Source: CAD feature listing. Evaluate the final solid. Frame: model axes, mm. A direction names the side the tool comes from. Give positions to 0.01 mm unless a question says otherwise; leave off trailing zeros. Order: outer loops, then holes, each group sorted by start corner. A loop starts at its lowest first (then second) coordinate and runs counter-clockwise, first axis right, second up. Notation, with made-up numbers: M 57,42.5 L 93,42.5 A30 ccw 93,70.5 Z; hole C -0.75,31.5 d9. An arc over 180 degrees is marked long. Use CSV: the item, a comma, the result in double quotes. Start each with the question number.
1. Reachability of faces 4 (the cylindrical face through (56.99, 1.52, -29.15)), 5 (the flat face through (-10, 1, -25)) from +Z, -Z, +X, -X, +Y, -Y: full face, straight path, thin tool, end or side. Return the list, or none.
2. Section query A-A, the plane y = 2.15. Return the cut outline in (x, z).
3. Line query: line 1 along X through (y, z) = (2.4, -17.5); line 2 along X through (y, z) = (2.35, -22); line 3 along Z through (x, y) = (-0.5, 1.25). Output: solid intervals per line, ascending. Write a range as [from, to].
4. Section query B-B, the plane x = -41. Return the cut outline in (y, z).
5. Mould query, pull axis X, two halves, no side actions, for faces 1 (the flat face through (0, 1, 32)), 2 (the flat face through (0, 1, -12)), 3 (the cylindrical face through (31.35, 1.48, 30.05)). Classes: released by +X, released by -X, zero draft, split by the parting line, or undercut.
6. Pin query (flat end, axial travel): P1, Ø1.5, axis at x = 29.5, z = 16, coming from the -Y side; P2, Ø0.9, axis at y = 1, z = -25, coming from the +X side; P3, Ø2.5, axis at x = 50, z = -22, coming from the +Y side. Return the tip coordinate at first contact, or that it passes through.
from build123d import *

# Parameters (mm, degrees)
SKETCH_1_W          = 120
SKETCH_1_H          = 64
EXTRUDE_1_DEPTH     = 3
SKETCH_2_R          = 1.5
CUT_EXTRUDE_1_DEPTH = 3
FILLET_1_R          = 10
SKETCH_3_W          = 20
SKETCH_3_H          = 20
CUT_EXTRUDE_2_DEPTH = 3
SKETCH_4_R          = 26
CUT_EXTRUDE_3_DEPTH = 3
FILLET_2_R          = 5
FILLET_3_R          = 10
FILLET_4_R          = 10
SKETCH_6_R          = 2.1
CUT_EXTRUDE_5_DEPTH = 6


with BuildPart() as part:
    # 草图1 → 凸台-拉伸1 (new body)
    with BuildSketch(Plane(origin=(0, 0, 0), x_dir=(1, 0, 0), z_dir=(0, 1, 0))):
        Rectangle(SKETCH_1_W, SKETCH_1_H)
    extrude(amount=EXTRUDE_1_DEPTH)

    # 草图2 → 切除-拉伸1 (cut)
    with BuildSketch(Plane(origin=(0, 3, 0), x_dir=(1, 0, 0), z_dir=(0, 1, 0))):
        with Locations(Location((-50, 22, 0), (0, 0, 270))):
            Circle(SKETCH_2_R)
        with Locations(Location((50, 22, 0), (0, 0, 90))):
            Circle(SKETCH_2_R)
    extrude(amount=-CUT_EXTRUDE_1_DEPTH, mode=Mode.SUBTRACT)

    # 圆角1
    fillet_1_edges = [part.edges().sort_by_distance(p)[0] for p in [
        (-60, 1.5, -32),
        (60, 1.5, -32),
    ]]
    fillet(fillet_1_edges, radius=FILLET_1_R)

    # 草图3 → 切除-拉伸2 (cut)
    with BuildSketch(Plane.XZ):
        with Locations((0, -22)):
            Rectangle(SKETCH_3_W, SKETCH_3_H)
    extrude(amount=-CUT_EXTRUDE_2_DEPTH, mode=Mode.SUBTRACT)

    # 草图4 → 切除-拉伸3 (cut)
    with BuildSketch(Plane.XZ):
        with Locations((-60, 32)):
            Circle(SKETCH_4_R)
        with Locations((60, 32)):
            Circle(SKETCH_4_R)
    extrude(amount=-CUT_EXTRUDE_3_DEPTH, mode=Mode.SUBTRACT)

    # 圆角2
    fillet_2_edges = [part.edges().sort_by_distance(p)[0] for p in [
        (-10, 1.5, -12),
        (10, 1.5, -12),
    ]]
    fillet(fillet_2_edges, radius=FILLET_2_R)

    # 圆角3
    fillet_3_edges = [part.edges().sort_by_distance(p)[0] for p in [
        (-60, 1.5, 6),
        (60, 1.5, 6),
    ]]
    fillet(fillet_3_edges, radius=FILLET_3_R)

    # 圆角4
    fillet_4_edges = [part.edges().sort_by_distance(p)[0] for p in [
        (-34, 1.5, 32),
        (34, 1.5, 32),
    ]]
    fillet(fillet_4_edges, radius=FILLET_4_R)

    # 草图6 → 切除-拉伸5 (cut)
    with BuildSketch(Plane(origin=(0, 3, 189.146349293), x_dir=(0, 0, 1), z_dir=(0, 1, 0))):
        with Locations((-209.45594255, -26.921391455)):
            Circle(SKETCH_6_R)
        with Locations((-167.762204108, 28.683304163)):
            Circle(SKETCH_6_R)
    extrude(amount=-CUT_EXTRUDE_5_DEPTH, mode=Mode.SUBTRACT)


solid = part.part
Result set:
1,face 4,"-Z, +X, +Y, -Y"
1,face 5,"-Z, +Y, -Y"
2,outline,"M -60,-22 A10 ccw -50,-32 L -10,-32 L -10,-17 A5 cw -5,-12 L 5,-12 A5 cw 10,-17 L 10,-32 L 50,-32 A10 ccw 60,-22 L 60,-2.58 A10 ccw 52.78,7.02 A26 cw 35.02,24.78 A10 ccw 25.42,32 L -25.42,32 A10 ccw -35.02,24.78 A26 cw -52.78,7.02 A10 ccw -60,-2.58 Z; hole C -50,-22 d3; hole C -26.92,-20.31 d4.2; hole C 28.68,21.38 d4.2; hole C 50,-22 d3"
3,line 1,"[-60, -10], [10, 60]"
3,line 2,"[-60, -51.5], [-48.5, -28.17], [-25.68, -10], [10, 48.5], [51.5, 60]"
3,line 3,"[-12, 32]"
4,outline,"M 0,-32 L 3,-32 L 3,14.25 L 0,14.25 Z"
5,face 1,"zero draft"
5,face 2,"undercut"
5,face 3,"released by +X"
6,P1,"y = 0"
6,P2,"x = 59.67"
6,P3,"through"
